Check sheet for the modelled part. Datum: model origin and axes. Units: mm. Give positions to 0.01 mm unless a question says otherwise; leave off trailing zeros. Loops run counter-clockwise (first coordinate to the right, second up) from the corner with the lowest first, then second, coordinate; pieces in that order, holes last. Notation, with made-up numbers: M -39.5,17 L -31.5,17 A21 cw -31.5,22 Z; hole C 0.5,61 d3. An arc over 180 degrees is marked long. Put each result on its own line as item: value. Start each with the question number.
Autodesk Inventor part; units mm, degrees
ref_plane "YZ Plane" through (0, 0, 0) normal (1, 0, 0) x (0, 1, 0)
ref_plane "XZ Plane" through (0, 0, 0) normal (0, 1, 0) x (-1, 0, 0)
ref_plane "XY Plane" through (0, 0, 0) normal (0, 0, 1) x (1, 0, 0)
sketch "Sketch1" plane through (0, 0, 0) normal (0, 0, 1) x (1, 0, 0)
  arc A0 (-9.525, 55.0553) -> (-15.875, 48.7053) centre (-9.525, 48.7053) ccw construction
  line L0 (-15.875, 19.05) -> (-15.875, 48.7053) construction
  line L1 (-15.875, 19.05) -> (15.875, 19.05) construction
  line L2 (15.875, 48.7053) -> (15.875, 19.05) construction
  arc A1 (15.875, 48.7053) -> (9.525, 55.0553) centre (9.525, 48.7053) ccw construction
  line L3 (-9.525, 55.0553) -> (9.525, 55.0553) construction
  circle A2 centre (9.525, 42.3553) radius 3.3782
  circle A3 centre (-9.525, 42.3553) radius 3.3782
  arc A4 (-256.923, 48.7053) -> (-263.273, 55.0553) centre (-263.273, 48.7053) ccw construction
  line L4 (-282.323, 55.0553) -> (-263.273, 55.0553) construction
  arc A5 (-282.323, 55.0553) -> (-288.673, 48.7053) centre (-282.323, 48.7053) ccw construction
  line L5 (-288.673, 19.05) -> (-288.673, 48.7053) construction
  line L6 (-288.673, 19.05) -> (-256.923, 19.05) construction
  line L7 (-256.923, 48.7053) -> (-256.923, 19.05) construction
  circle A6 centre (-263.273, 42.3553) radius 3.3782
  circle A7 centre (-282.323, 42.3553) radius 3.3782
  line L8 (-288.673, 55.0553) -> (15.875, 55.0553)
  line L9 (-288.673, 29.6553) -> (15.875, 29.6553)
  line L10 (-288.673, 29.6553) -> (-288.673, 55.0553)
  line L11 (15.875, 29.6553) -> (15.875, 55.0553)
  line L12 (-288.673, 42.3553) -> (15.875, 42.3553) construction
  circle A8 centre (-237.873, 42.3553) radius 7.9375
  circle A9 centre (-208.8804, 42.3553) radius 7.9375
  circle A10 centre (-179.8879, 42.3553) radius 7.9375
  circle A11 centre (-150.8953, 42.3553) radius 7.9375
  circle A12 centre (-121.9027, 42.3553) radius 7.9375
  circle A13 centre (-92.9101, 42.3553) radius 7.9375
  circle A14 centre (-63.9176, 42.3553) radius 7.9375
  circle A15 centre (-34.925, 42.3553) radius 7.9375
  point P0 (0, 0)
  dimension "d1" = 25.4
  dimension "d2" = 12.7
  dimension "d33" = 15.875
  dimension "d35" = 304.548
  dimension "d36" = 50.8
  dimension "d39" = 28.9926
extrude "Plate1" add sketch "Sketch1" along normal blind 3.048
fillet "Corner Round1" radius 6.35 4 edges at (-288.673, 29.6553, 1.524) (-288.673, 55.0553, 1.524) (15.875, 29.6553, 1.524) (15.875, 55.0553, 1.524)
equation "\"d39\" = -0.285714 * d36 + 0.142857 * d35"
equation "\"BendRadius\" = Thickness"
equation "\"BendReliefWidth\" = Thickness"
equation "\"BendReliefDepth\" = 0.5 * Thickness"
equation "\"CornerReliefSize\" = 4 * Thickness"
equation "\"MinimumRemnant\" = 2 * Thickness"
equation "\"TransitionRadius\" = BendRadius"
equation "\"JacobiRadiusSize\" = BendRadius"
equation "\"GapSize\" = Thickness"
equation "\"d3\" = BendRadius"
properties part number "V5 Shooter Frame Channel P7" material "Aluminum-6061"
Q1. Thickness scan on line 1 along Y through (x, z) = (-68, 1.4); line 2 along Y through (x, z) = (-237.5, 1.2); line 3 along X through (y, z) = (33, 1.05). Record the ranges inside material, lowest first. Write a range as [from, to].
Q2. Section check C-C, the plane x = -181. Record the cut outline in (y, z).
Q3. Section check B-B, the plane z = 2.05. Give the number of separate pieces and of enclosed holes in the cut face, then the cut area to 3 significant figures.
Q4. Mould release check, pull along Y, two halves, no side actions. Record for faces 1 (the face through (-287, 53, 2)), 2 (the face through (-172.556, 45.395, 1.503)), 3 (the face through (-286.86, 31.56, 1.55)): pulls with the +Y half, pulls with the -Y half, needs draft (parallel to the pull), parting line crosses it, or undercut.
Q5. Depth check by flat-ended pin: P1, Ø1.5, axis at y = 34, z = 1.5, coming from the +X side. Enter the tip coordinate at first touch or a pass-through.
Q6. Section check A-A, the plane x = -94. Record the cut outline in (y, z).
Found:
1. line 1: y = [29.66, 35.55], [49.16, 55.06]
1. line 2: y = [29.66, 34.43], [50.28, 55.06]
1. line 3: x = [-287.92, 15.12]
2. outline: M 29.66,0 L 34.5,0 L 34.5,3.05 L 29.66,3.05 Z; M 50.21,0 L 55.06,0 L 55.06,3.05 L 50.21,3.05 Z
3. separate pieces: 1
3. enclosed holes: 12
3. area: 5,970 mm^2
4. face 1: pulls with the +Y half
4. face 2: undercut
4. face 3: pulls with the -Y half
5. P1: stops at x = 15.75
6. outline: M 29.66,0 L 34.49,0 L 34.49,3.05 L 29.66,3.05 Z; M 50.22,0 L 55.06,0 L 55.06,3.05 L 50.22,3.05 Z
